```python
from build123d import *

# Parameters (mm, degrees)
SKETCH2_R          = 0.5
CUT_EXTRUDE1_DEPTH = 5
CHAMFER1_SIZE      = 0.5


with BuildPart() as part:
    # Sketch1 → Revolve1 (revolve)
    with BuildSketch(Plane(origin=(0, 0, 0), x_dir=(0, 0, -1), z_dir=(1, 0, 0)), mode=Mode.PRIVATE) as revolve1_sk:
        with BuildLine():
            Line((0, 1.994594595), (39, 1.994594595))
            Line((39, 1.994594595), (39, 3))
            ThreePointArc((39, 3), (41.121320344, 2.121320344), (42, 0))
            Line((42, 0), (0, 0))
            Line((0, 0), (0, 1.994594595))
        make_face()
    revolve(revolve1_sk.sketch.rotate(Axis((0, 0, 0), (0, 0, -1)), 90), axis=Axis((0, 0, 0), (0, 0, -1)))

    # Sketch2 → Cut-Extrude1 (cut, symmetric)
    with BuildSketch(Plane(origin=(0, 0, 0), x_dir=(0, 0, -1), z_dir=(1, 0, 0))):
        with Locations((2, 0)):
            Circle(SKETCH2_R)
    extrude(amount=CUT_EXTRUDE1_DEPTH, both=True, mode=Mode.SUBTRACT)

    # Chamfer1
    chamfer1_edges = [part.edges().sort_by_distance(p)[0] for p in [
        (-1.994594595, 0, 0),
    ]]
    chamfer(chamfer1_edges, length=CHAMFER1_SIZE)


solid = part.part
```
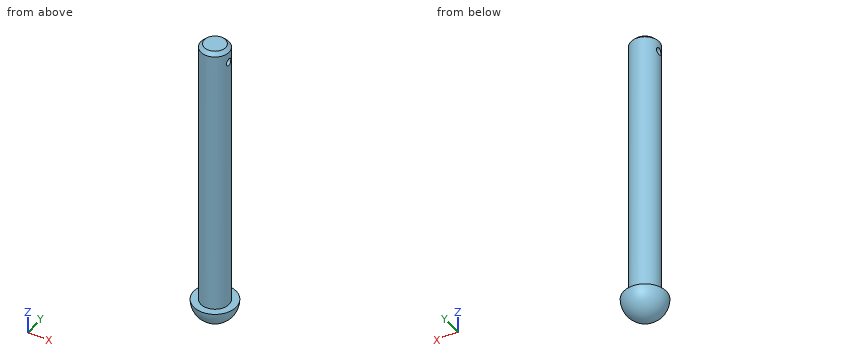
Design review of the part built by this model. Coordinates are the model's own, in mm. Give positions to 0.01 mm unless a question says otherwise; leave off trailing zeros. Order: outer loops, then holes, each group sorted by start corner. A loop starts at its lowest first (then second) coordinate and runs counter-clockwise, first axis right, second up. Notation, with made-up numbers: (61, -39.75) -> (78, -39.75) arc R24 ccw to (78, -20.75) -> close; hole circle Ø11 at (29.25, -15). An arc over 180 degrees is marked (long way). Write each question's results on one line, items separated by ' | '. Start each with the question number.
Q1. Add section C-C on z = -36. Give the boundary of the cut face in (x, y).
Q2. Add section D-D on z = -2. Give the boundary of the cut face in (x, y), and give its area (3 significant figures).
Q3. Add section A-A on y = 0. Give the boundary of the cut face in (x, z), and give its area (3 significant figures).
Q4. Add section B-B on x = 0. Give the boundary of the cut face in (y, z).
Q5. Wall thickness on L1, parallel to Z at x = -0.55, y = 0; L2, parallel to Y at x = -0.85, z = -2; L3, parallel to Y at x = 0.7, z = -2: over which ranges is each line inside the solid? List them lowest first. Write a range as from..to.
Q6. For pin 1 (2 mm diameter, centred on x = 1.5, y = -1.5, fed in from +Z); pin 2 (1.5 mm diameter, centred on y = 0, z = -35.5, fed in from -X); pin 3 (2 mm diameter, centred on x = 0, z = -31.5, fed in from -Y); pin 4 (2 mm diameter, centred on y = -2, z = -9.5, fed in from +X), all flat-tipped, find the tip position at first contact; note any pin that passes through.
Found:
1) outline: circle Ø3.99 at (0, 0)
2) outline: (-1.93, -0.5) arc R1.99 ccw to (1.93, -0.5) -> close; (-1.93, 0.5) -> (1.93, 0.5) arc R1.99 ccw to start | area: 8.55 mm2
3) outline: (-3, -39) arc R3 ccw to (3, -39) -> (1.99, -39) -> (1.99, -2.5) -> (-1.99, -2.5) -> (-1.99, -39) -> close; (-1.99, -1.5) -> (1.99, -1.5) -> (1.99, -0.5) -> (1.49, 0) -> (-1.49, 0) -> (-1.99, -0.5) -> close | area: 165 mm2
4) outline: (-3, -39) arc R3 ccw to (3, -39) -> (1.99, -39) -> (1.99, -0.5) -> (1.49, 0) -> (-1.49, 0) -> (-1.99, -0.5) -> (-1.99, -39) -> close; hole circle Ø1 at (0, -2)
5) L1: z = -41.95..-2.5, -1.5..0 | L2: y = -1.8..-0.5, 0.5..1.8 | L3: y = -1.87..-0.5, 0.5..1.87
6) pin 1: stops at z = 0 | pin 2: stops at x = -1.99 | pin 3: stops at y = -1.99 | pin 4: stops at x = 1.73
